Check sheet for the modelled part. Datum: model origin and axes. Units: mm. Coordinates: 2 decimals unless noted, no trailing zeros. Order: outer loops, then holes, each group sorted by start corner. A loop starts at its lowest first (then second) coordinate and runs counter-clockwise, first axis right, second up.
from build123d import *

# Parameters (mm, degrees)
EXTRUDE_1_DEPTH     = 5
SKETCH_2_R          = 2.1
CUT_EXTRUDE_1_DEPTH = 6
FILLET_1_R          = 5
SKETCH_3_R          = 2.5
CUT_EXTRUDE_2_DEPTH = 6
SKETCH_4_R          = 2.1
CUT_EXTRUDE_3_DEPTH = 6
SKETCH_5_W          = 160
SKETCH_5_H          = 66.889435481
CUT_EXTRUDE_4_DEPTH = 6
FILLET_2_R          = 5
CUT_EXTRUDE_5_DEPTH = 6


with BuildPart() as part:
    # 草图1 → 凸台-拉伸1 (new body)
    with BuildSketch(Plane(origin=(0, 0, 0), x_dir=(1, 0, 0), z_dir=(0, 1, 0))):
        Polygon((-180, 180), (-180, 103), (-80, 103), (-80, 180), (80, 180), (80, 103), (180, 103), (180, 180), (210, 180), (210, -180), (180, -180), (180, -103), (80, -103), (80, -180), (-80, -180), (-80, -103), (-180, -103), (-180, -180), (-210, -180), (-210, 180), align=None)
    extrude(amount=EXTRUDE_1_DEPTH)

    # 草图2 → 切除-拉伸1 (cut, through all)
    with BuildSketch(Plane(origin=(0, 5, 0), x_dir=(1, 0, 0), z_dir=(0, 1, 0))):
        with Locations((115, -88.5)):
            Circle(SKETCH_2_R)
        with Locations((145, -88.5)):
            Circle(SKETCH_2_R)
        with Locations((130, -95.5)):
            Circle(SKETCH_2_R)
        with Locations((130, 95.5)):
            Circle(SKETCH_2_R)
        with Locations((145, 88.5)):
            Circle(SKETCH_2_R)
        with Locations((115, 88.5)):
            Circle(SKETCH_2_R)
        with Locations((-115, 88.5)):
            Circle(SKETCH_2_R)
        with Locations((-145, 88.5)):
            Circle(SKETCH_2_R)
        with Locations((-130, 95.5)):
            Circle(SKETCH_2_R)
        with Locations((-130, -95.5)):
            Circle(SKETCH_2_R)
        with Locations((-145, -88.5)):
            Circle(SKETCH_2_R)
        with Locations((-115, -88.5)):
            Circle(SKETCH_2_R)
    extrude(amount=-CUT_EXTRUDE_1_DEPTH, mode=Mode.SUBTRACT)

    # 圆角1
    fillet_1_edges = [part.edges().sort_by_distance(p)[0] for p in [
        (180, 2.5, 180),
        (80, 2.5, 180),
        (-80, 2.5, 180),
        (-180, 2.5, 180),
        (-180, 2.5, -180),
        (-80, 2.5, -180),
        (80, 2.5, -180),
        (180, 2.5, -180),
    ]]
    fillet(fillet_1_edges, radius=FILLET_1_R)

    # 草图3 → 切除-拉伸2 (cut, through all)
    with BuildSketch(Plane.XZ):
        with Locations((84.75, 31.75)):
            Circle(SKETCH_3_R)
        with Locations((84.75, -31.75)):
            Circle(SKETCH_3_R)
        with Locations((171.25, 31.75)):
            Circle(SKETCH_3_R)
        with Locations((171.25, -31.75)):
            Circle(SKETCH_3_R)
        with Locations((-171.25, -31.75)):
            Circle(SKETCH_3_R)
        with Locations((-171.25, 31.75)):
            Circle(SKETCH_3_R)
        with Locations((-84.75, -31.75)):
            Circle(SKETCH_3_R)
        with Locations((-84.75, 31.75)):
            Circle(SKETCH_3_R)
    extrude(amount=-CUT_EXTRUDE_2_DEPTH, mode=Mode.SUBTRACT)

    # 草图4 → 切除-拉伸3 (cut, through all)
    with BuildSketch(Plane.XZ):
        with Locations((-125, 0)):
            Circle(SKETCH_4_R)
        with Locations((125, 0)):
            Circle(SKETCH_4_R)
        with Locations((0, 10)):
            Circle(SKETCH_4_R)
        with Locations((0, -10)):
            Circle(SKETCH_4_R)
    extrude(amount=-CUT_EXTRUDE_3_DEPTH, mode=Mode.SUBTRACT)

    # 草图5 → 切除-拉伸4 (cut, through all)
    with BuildSketch(Plane(origin=(0, 5, 0), x_dir=(1, 0, 0), z_dir=(0, 1, 0))):
        with Locations((0, -172.444717741)):
            Rectangle(SKETCH_5_W, SKETCH_5_H)
        Polygon((80, 139), (-80, 139), (-80, 214.558464343), (80, 221.06023599), align=None)
    extrude(amount=-CUT_EXTRUDE_4_DEPTH, mode=Mode.SUBTRACT)

    # 圆角2
    fillet_2_edges = [part.edges().sort_by_distance(p)[0] for p in [
        (-80, 2.5, 139),
        (80, 2.5, 139),
        (80, 2.5, -139),
        (-80, 2.5, -139),
    ]]
    fillet(fillet_2_edges, radius=FILLET_2_R)

    # 草图6 → 切除-拉伸5 (cut, through all)
    with BuildSketch(Plane(origin=(0, 5, 0), x_dir=(1, 0, 0), z_dir=(0, 1, 0))):
        with BuildLine():
            Line((-60, 123), (60, 123))
            ThreePointArc((60, 123), (62.1, 120.9), (60, 118.8))
            Line((60, 118.8), (-60, 118.8))
            ThreePointArc((-60, 118.8), (-62.1, 120.9), (-60, 123))
        make_face()
        with BuildLine():
            Line((-40, 108.8), (40, 108.8))
            ThreePointArc((40, 108.8), (42.1, 106.7), (40, 104.6))
            Line((40, 104.6), (-40, 104.6))
            ThreePointArc((-40, 104.6), (-42.1, 106.7), (-40, 108.8))
        make_face()
        with BuildLine():
            Line((-62.1, 110), (-62.1, 20))
            ThreePointArc((-62.1, 20), (-60, 17.9), (-57.9, 20))
            Line((-57.9, 20), (-57.9, 110))
            ThreePointArc((-57.9, 110), (-60, 112.1), (-62.1, 110))
        make_face()
        with BuildLine():
            Line((-40, 94.6), (40, 94.6))
            ThreePointArc((40, 94.6), (42.1, 92.5), (40, 90.4))
            Line((40, 90.4), (-40, 90.4))
            ThreePointArc((-40, 90.4), (-42.1, 92.5), (-40, 94.6))
        make_face()
        with BuildLine():
            Line((62.1, 110), (62.1, 20))
            ThreePointArc((62.1, 20), (60, 17.9), (57.9, 20))
            Line((57.9, 20), (57.9, 110))
            ThreePointArc((57.9, 110), (60, 112.1), (62.1, 110))
        make_face()
        with BuildLine():
            Line((-40, 64.2), (40, 64.2))
            ThreePointArc((40, 64.2), (42.1, 62.1), (40, 60))
            Line((40, 60), (-40, 60))
            ThreePointArc((-40, 60), (-42.1, 62.1), (-40, 64.2))
        make_face()
        with BuildLine():
            Line((-40, 50), (40, 50))
            ThreePointArc((40, 50), (42.1, 47.9), (40, 45.8))
            Line((40, 45.8), (-40, 45.8))
            ThreePointArc((-40, 45.8), (-42.1, 47.9), (-40, 50))
        make_face()
        with BuildLine():
            Line((40, -60), (-40, -60))
            ThreePointArc((-40, -60), (-42.1, -62.1), (-40, -64.2))
            Line((-40, -64.2), (40, -64.2))
            ThreePointArc((40, -64.2), (42.1, -62.1), (40, -60))
        make_face()
        with BuildLine():
            Line((40, -45.8), (-40, -45.8))
            ThreePointArc((-40, -45.8), (-42.1, -47.9), (-40, -50))
            Line((-40, -50), (40, -50))
            ThreePointArc((40, -50), (42.1, -47.9), (40, -45.8))
        make_face()
        with BuildLine():
            Line((-57.9, -110), (-57.9, -20))
            ThreePointArc((-57.9, -20), (-60, -17.9), (-62.1, -20))
            Line((-62.1, -20), (-62.1, -110))
            ThreePointArc((-62.1, -110), (-60, -112.1), (-57.9, -110))
        make_face()
        with BuildLine():
            Line((57.9, -20), (57.9, -110))
            ThreePointArc((57.9, -110), (60, -112.1), (62.1, -110))
            Line((62.1, -110), (62.1, -20))
            ThreePointArc((62.1, -20), (60, -17.9), (57.9, -20))
        make_face()
        with BuildLine():
            Line((40, -90.4), (-40, -90.4))
            ThreePointArc((-40, -90.4), (-42.1, -92.5), (-40, -94.6))
            Line((-40, -94.6), (40, -94.6))
            ThreePointArc((40, -94.6), (42.1, -92.5), (40, -90.4))
        make_face()
        with BuildLine():
            Line((40, -104.6), (-40, -104.6))
            ThreePointArc((-40, -104.6), (-42.1, -106.7), (-40, -108.8))
            Line((-40, -108.8), (40, -108.8))
            ThreePointArc((40, -108.8), (42.1, -106.7), (40, -104.6))
        make_face()
        with BuildLine():
            Line((60, -118.8), (-60, -118.8))
            ThreePointArc((-60, -118.8), (-62.1, -120.9), (-60, -123))
            Line((-60, -123), (60, -123))
            ThreePointArc((60, -123), (62.1, -120.9), (60, -118.8))
        make_face()
    extrude(amount=-CUT_EXTRUDE_5_DEPTH, mode=Mode.SUBTRACT)


solid = part.part
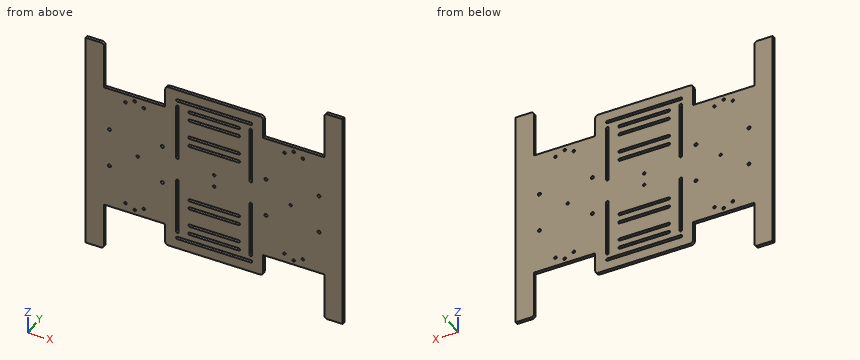
(1) Go/stop test with flat-tipped pins: P1, Ø1.5, axis at x = 4, y = 1.5, coming from the -Z side; P2, Ø1.5, axis at x = -12.5, y = 3.5, coming from the +Z side. Record where each tip stops, or that it passes through.
Filled in:
P1: stops at z = -139
P2: stops at z = 139
(2) Cross-section at A-A (x = -28). Count the separate pieces of the cut face and the enclosed holes in it, and give its area (3 significant figures).
Filled in:
separate pieces: 11
enclosed holes: 0
area: 1,180 mm2
(3) Cross-section at C-C (x = 93.5). Enter the section's corners in (y, z), and give its area (3 significant figures).
Filled in:
outline: (0, -103) - (5, -103) - (5, 103) - (0, 103) - close
area: 1,030 mm2
(4) Thickness scan on probe 1 along Z at (x, y) = (171.25, 3.6); probe 2 along Z at (x, y) = (-130, 3.95); probe 3 along X at (y, z) = (1.6, -132). Record the ranges inside material, lowest first.
Filled in:
probe 1: z = -103 to -34.25, -29.25 to 29.25, 34.25 to 103
probe 2: z = -103 to -97.6, -93.4 to 93.4, 97.6 to 103
probe 3: x = -210 to -180, -80 to 80, 180 to 210
